Design review of the part built by this model. Coordinates are the model's own, in mm. Coordinates: 2 decimals unless noted, no trailing zeros. Loops run counter-clockwise (first coordinate to the right, second up) from the corner with the lowest first, then second, coordinate; pieces in that order, holes last. Notation, with made-up numbers: M 76.25,19 L 89.25,19 A19 cw 89.25,53 Z; hole C -29.5,35.25 d2. An arc over 180 degrees is marked long. One line per item, written item: value.
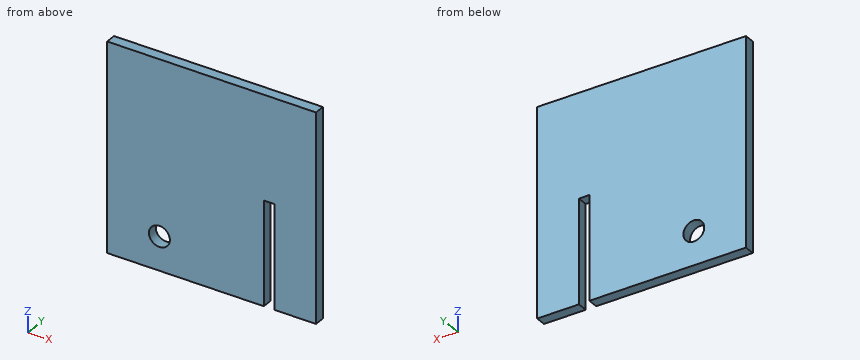
```python
from build123d import *

# Parameters (mm, degrees)
SKETCH1_W               = 254
SKETCH1_H               = 254
BOSS_EXTRUDE1_DEPTH     = 6.35
CAVITY1_START           = -6.35
CAVITY1_OUTLINE_R       = 12.7
CAVITY1_DEPTH           = 12.7
CUT_EXTRUDE1_DEPTH      = 285.051619429
CUT_EXTRUDE1_DEPTH_BACK = 285.051619429
SKETCH2_W               = 12.7
SKETCH2_H               = 127


# Read off the part's stored shape, not the designer's step: Cavity1
with BuildPart() as part:
    # Sketch1 → Boss-Extrude1 (new, symmetric)
    with BuildSketch(Plane(origin=(0, 0, 0), x_dir=(1, 0, 0), z_dir=(0, 1, 0))):
        with Locations((0, 127)):
            Rectangle(SKETCH1_W, SKETCH1_H)
    extrude(amount=BOSS_EXTRUDE1_DEPTH, both=True)

    # Cavity1 outline → Cavity1 (cut)
    with BuildSketch(Plane(origin=(0, 0, 0), x_dir=(1, 0, 0), z_dir=(0, 1, 0)).offset(CAVITY1_START)):
        with Locations((-63.5, 212.75)):
            Circle(CAVITY1_OUTLINE_R)
    extrude(amount=CAVITY1_DEPTH, mode=Mode.SUBTRACT)

    # Sketch2 → Cut-Extrude1 (cut, two sides: drawn at the far end of the back side and taken through both)
    with BuildSketch(Plane(origin=(0, 0, 0), x_dir=(1, 0, 0), z_dir=(0, 1, 0)).offset(-CUT_EXTRUDE1_DEPTH_BACK)):
        with Locations((69.85, 190.5)):
            Rectangle(SKETCH2_W, SKETCH2_H)
    extrude(amount=CUT_EXTRUDE1_DEPTH + CUT_EXTRUDE1_DEPTH_BACK, mode=Mode.SUBTRACT)


solid = part.part
```
(1) To check wall thickness, follow line 1 along X through (y, z) = (3.5, -212.75); line 2 along Z through (x, y) = (-63.5, 1.5); line 3 along X through (y, z) = (-3.5, -145). State the ranges of each line that lie inside material, in increasing order. Write a range as [from, to].
Reply:
line 1: x = [-127, -76.2], [-50.8, 63.5], [76.2, 127]
line 2: z = [-254, -225.45], [-200.05, 0]
line 3: x = [-127, 63.5], [76.2, 127]
(2) Insertion check: pin 1 (20.5 mm diameter, centred on x = -63.5, z = -212.75, fed in from +Y). The pin has a flat end and moves straight along its axis. Give the tip position at first contact, or say it passes through.
Reply:
pin 1: passes through
(3) We need section B-B on z = -212.75. State the section outline as (x, y) points.
Reply:
outline: M -127,-6.35 L -76.2,-6.35 L -76.2,6.35 L -127,6.35 Z; M -50.8,-6.35 L 63.5,-6.35 L 63.5,6.35 L -50.8,6.35 Z; M 76.2,-6.35 L 127,-6.35 L 127,6.35 L 76.2,6.35 Z
(4) We need section A-A on x = -63.5. State the section outline as (y, z) points, then the cut area to 3 significant figures.
Reply:
outline: M -6.35,-254 L 6.35,-254 L 6.35,-225.45 L -6.35,-225.45 Z; M -6.35,-200.05 L 6.35,-200.05 L 6.35,0 L -6.35,0 Z
area: 2,900 mm2
(5) We need section C-C on y = -3.25. State the section outline as (x, z) points.
Reply:
outline: M -127,-254 L 63.5,-254 L 63.5,-127 L 76.2,-127 L 76.2,-254 L 127,-254 L 127,0 L -127,0 Z; hole C -63.5,-212.75 d25.4
